```python
from build123d import *

# Parameters (mm, degrees)
F0_R      = 27.5
F1_DEPTH  = 5
F2_R      = 5
F3_DEPTH  = 5
F4_R      = 1.85
F5_DEPTH  = 10
F6_R      = 3
F6_R_2    = 1.85
F7_DEPTH  = 1.5
F9_DEPTH  = 5
F10_R     = 31.5
F10_R_2   = 27.5
F10_R_3   = 1.85
F11_DEPTH = 1
F8_R      = 1.3
F8_R_2    = 2.15
F12_DEPTH = 6


with BuildPart() as f1:
    # F0 (on Top) → F1 (new body)
    with BuildSketch(Plane.XY):
        Circle(F0_R)
    extrude(amount=F1_DEPTH)

    # F2 (on face) → F3 (join)
    with BuildSketch(Plane.XY.offset(5)):
        Circle(F2_R)
    extrude(amount=F3_DEPTH)

    # F4 (on face) → F5 (cut, through all)
    with BuildSketch(Plane.XY.offset(10)):
        Circle(F4_R)
    extrude(amount=-F5_DEPTH, mode=Mode.SUBTRACT)

    # F6 (on face) → F7 (join)
    with BuildSketch(Plane.XY.offset(10)):
        Circle(F6_R)
        Circle(F6_R_2, mode=Mode.SUBTRACT)
    extrude(amount=F7_DEPTH)

    # F8 (on face) → F9 (cut, through all)
    with BuildSketch(Plane.XY.offset(5)):
        with BuildLine():
            Line((5.5901699437, 5), (24.4948974278, 5))
            ThreePointArc((24.4948974278, 5), (17.6776695297, 17.6776695297), (5, 24.4948974278))
            Line((5, 24.4948974278), (5, 5.5901699437))
            ThreePointArc((5, 5.5901699437), (5.3033008589, 5.3033008589), (5.5901699437, 5))
        make_face()
        with BuildLine():
            Line((-5, 5.5901699437), (-5, 24.4948974278))
            ThreePointArc((-5, 24.4948974278), (-17.6776695297, 17.6776695297), (-24.4948974278, 5))
            Line((-24.4948974278, 5), (-5.5901699437, 5))
            ThreePointArc((-5.5901699437, 5), (-5.3033008589, 5.3033008589), (-5, 5.5901699437))
        make_face()
        with BuildLine():
            ThreePointArc((-24.4948974278, -5), (-17.6776695297, -17.6776695297), (-5, -24.4948974278))
            Line((-5, -24.4948974278), (-5, -5.5901699437))
            ThreePointArc((-5, -5.5901699437), (-5.3033008589, -5.3033008589), (-5.5901699437, -5))
            Line((-5.5901699437, -5), (-24.4948974278, -5))
        make_face()
        with BuildLine():
            ThreePointArc((5, -24.4948974278), (17.6776695297, -17.6776695297), (24.4948974278, -5))
            Line((24.4948974278, -5), (5.5901699437, -5))
            ThreePointArc((5.5901699437, -5), (5.3033008589, -5.3033008589), (5, -5.5901699437))
            Line((5, -5.5901699437), (5, -24.4948974278))
        make_face()
    extrude(amount=-F9_DEPTH, mode=Mode.SUBTRACT)

    # F10 (on face) → F11 (join)
    with BuildSketch(Plane(origin=(0, 0, 0), x_dir=(1, 0, 0), z_dir=(0, 0, -1))):
        Circle(F10_R)
        Circle(F10_R_2, mode=Mode.SUBTRACT)
        Circle(F10_R_2)
        with BuildLine():
            ThreePointArc((-5, -24.4948974278), (-17.6776695297, -17.6776695297), (-24.4948974278, -5))
            Line((-24.4948974278, -5), (-5.5901699437, -5))
            ThreePointArc((-5.5901699437, -5), (-5.3033008589, -5.3033008589), (-5, -5.5901699437))
            Line((-5, -5.5901699437), (-5, -24.4948974278))
        make_face(mode=Mode.SUBTRACT)
        with BuildLine():
            ThreePointArc((24.4948974278, -5), (17.6776695297, -17.6776695297), (5, -24.4948974278))
            Line((5, -24.4948974278), (5, -5.5901699437))
            ThreePointArc((5, -5.5901699437), (5.3033008589, -5.3033008589), (5.5901699437, -5))
            Line((5.5901699437, -5), (24.4948974278, -5))
        make_face(mode=Mode.SUBTRACT)
        with BuildLine():
            ThreePointArc((-24.4948974278, 5), (-17.6776695297, 17.6776695297), (-5, 24.4948974278))
            Line((-5, 24.4948974278), (-5, 5.5901699437))
            ThreePointArc((-5, 5.5901699437), (-5.3033008589, 5.3033008589), (-5.5901699437, 5))
            Line((-5.5901699437, 5), (-24.4948974278, 5))
        make_face(mode=Mode.SUBTRACT)
        Circle(F10_R_3, mode=Mode.SUBTRACT)
        with BuildLine():
            ThreePointArc((5, 24.4948974278), (17.6776695297, 17.6776695297), (24.4948974278, 5))
            Line((24.4948974278, 5), (5.5901699437, 5))
            ThreePointArc((5.5901699437, 5), (5.3033008589, 5.3033008589), (5, 5.5901699437))
            Line((5, 5.5901699437), (5, 24.4948974278))
        make_face(mode=Mode.SUBTRACT)
    extrude(amount=F11_DEPTH)

    # F8 (on face) → F12 (cut, through all)
    with BuildSketch(Plane.XY.offset(5)):
        with Locations((-12, 0)):
            Circle(F8_R)
        with Locations((0, -15.5)):
            Circle(F8_R_2)
        with Locations((12, 0)):
            Circle(F8_R)
        with Locations((0, 15.5)):
            Circle(F8_R_2)
    extrude(amount=-F12_DEPTH, mode=Mode.SUBTRACT)


solid = f1.part
```
Read the model definition and answer for the solid it produces. Units are mm, in the model's axes. A direction names the side the tool comes from. Coordinates: 2 decimals unless noted, no trailing zeros. Write each loop counter-clockwise with the first axis right and the second up, starting at its lowest first coordinate (ties: lowest second). Pieces come first, ordered by that corner, then holes. Notation, with made-up numbers: (4, 17.25) -> (47, 17.25) arc R19 cw to (47, 48.25) -> close; hole circle Ø10 at (14.5, -30). An arc over 180 degrees is marked (long way). Return JSON: item names as keys, results as strings.
1. Determine the mould class of faces 1 (the face through (4, -4, 5)), 2 (the face through (5, -15, 2)), 3 (the face through (-4.101, -31.232, -0.493)) for opening direction X: pulls with the +X half, pulls with the -X half, needs draft (parallel to the pull), parting line crosses it, or undercut.
Found:
{"face 1": "needs draft", "face 2": "undercut", "face 3": "parting line crosses it"}
2. A cutting plane is placed at C-C (y = 0). Determine the outline of the cut face in (x, z), and give its area (3 significant figures).
Found:
{"outline": "(-31.5, -1) -> (-13.3, -1) -> (-13.3, 5) -> (-27.5, 5) -> (-27.5, 0) -> (-31.5, 0) -> close; (-10.7, -1) -> (-1.85, -1) -> (-1.85, 11.5) -> (-3, 11.5) -> (-3, 10) -> (-5, 10) -> (-5, 5) -> (-10.7, 5) -> close; (1.85, -1) -> (10.7, -1) -> (10.7, 5) -> (5, 5) -> (5, 10) -> (3, 10) -> (3, 11.5) -> (1.85, 11.5) -> close; (13.3, -1) -> (31.5, -1) -> (31.5, 0) -> (27.5, 0) -> (27.5, 5) -> (13.3, 5) -> close", "area": "320 mm2"}
3. Each of these flat-tipped pins is pushed along its axis until it touches: P1, Ø1.8, axis at x = 15.5, z = 2, coming from the -Y side; P2, Ø2.5, axis at x = 0, y = 15.5, coming from the -Z side; P3, Ø5, axis at x = -19, z = 2, coming from the -Y side; P4, Ø1.8, axis at x = 18, z = 2, coming from the +Y side. Where does it stop, or does it pass through?
Found:
{"P1": "y = -23.3", "P2": "through", "P3": "y = -26.19", "P4": "y = 21.54"}
4. A tool of negligible diameter and unlimited length cuts with its end or side. For faces 4 (the face through (0, 28, 0)), 5 (the face through (-5, -15, 2)), 6 (the face through (1, -2, 11.5)), from which of +Z, -Z, +X, -X, +Y, -Y can it reach the whole face along a straight path? Write none if from no direction.
Found:
{"face 4": "+Z", "face 5": "+Z, -Z", "face 6": "+Z, +X, -X, +Y, -Y"}
5. Find the intervals of material crossed by line 1 along Y through (x, z) = (0, 1.1); line 2 along X through (y, z) = (-22, 1); line 3 along Y through (x, z) = (0, 9.25), in increasing order. Write a range as from..to.
Found:
{"line 1": "-27.5..-17.65, -13.35..-1.85, 1.85..13.35, 17.65..27.5", "line 2": "-16.5..-11.87, -5..5, 11.87..16.5", "line 3": "-5..-1.85, 1.85..5"}
6. A cutting plane is placed at A-A (x = 0). Determine the outline of the cut face in (y, z), and give its area (3 significant figures).
Found:
{"outline": "(-31.5, -1) -> (-17.65, -1) -> (-17.65, 5) -> (-27.5, 5) -> (-27.5, 0) -> (-31.5, 0) -> close; (-13.35, -1) -> (-1.85, -1) -> (-1.85, 11.5) -> (-3, 11.5) -> (-3, 10) -> (-5, 10) -> (-5, 5) -> (-13.35, 5) -> close; (1.85, -1) -> (13.35, -1) -> (13.35, 5) -> (5, 5) -> (5, 10) -> (3, 10) -> (3, 11.5) -> (1.85, 11.5) -> close; (17.65, -1) -> (31.5, -1) -> (31.5, 0) -> (27.5, 0) -> (27.5, 5) -> (17.65, 5) -> close", "area": "299 mm2"}
7. A cutting plane is placed at B-B (z = 3.25). Give the number of separate pieces and of enclosed holes in the cut face, and give its area (3 significant figures).
Found:
{"separate pieces": "1", "enclosed holes": "9", "area": "1,260 mm2"}
8. A cutting plane is placed at D-D (y = 8.5). Determine the outline of the cut face in (x, z), and give its area (3 significant figures).
Found:
{"outline": "(-30.33, -1) -> (-23.51, -1) -> (-23.51, 5) -> (-26.15, 5) -> (-26.15, 0) -> (-30.33, 0) -> close; (-5, -1) -> (5, -1) -> (5, 5) -> (-5, 5) -> close; (23.51, -1) -> (30.33, -1) -> (30.33, 0) -> (26.15, 0) -> (26.15, 5) -> (23.51, 5) -> close", "area": "100 mm2"}
